Study the drawing (mm; zero at the part's minimum x, y, z) and answer. Coordinates: 2 decimals unless noted, no trailing zeros. Loops run counter-clockwise (first coordinate to the right, second up) from the corner with the lowest first, then second, coordinate; pieces in that order, holes last. Notation, with made-up numbers: (-6, 82) - (52, 82) arc R6 ccw to (52, 92) - close; hole circle Ø11 at (78.25, -37). An arc over 180 degrees is marked (long way). Write each question's results on one line, items separated by ' | '. Start each with the question number.
(1) Find section C-C on z = 2.55. Determine the outline of the cut face in (x, y), then the cut area to 3 significant figures.
(2) Consider line 1 (Y direction, x = 55, z = 1.4); line 2 (X direction, y = 27, z = 4.55); line 3 (Z direction, x = 57.5, y = 53). Determine where each line is inside the solid, lowest interval first. Write a range as from..to.
(3) Find section A-A on y = 16. Determine the outline of the cut face in (x, z), then the cut area to 3 significant figures.
(4) Find section D-D on x = 26. Determine the outline of the cut face in (y, z).
(5) Find section B-B on x = 4.5. Determine the outline of the cut face in (y, z), then the cut area to 3 significant figures.
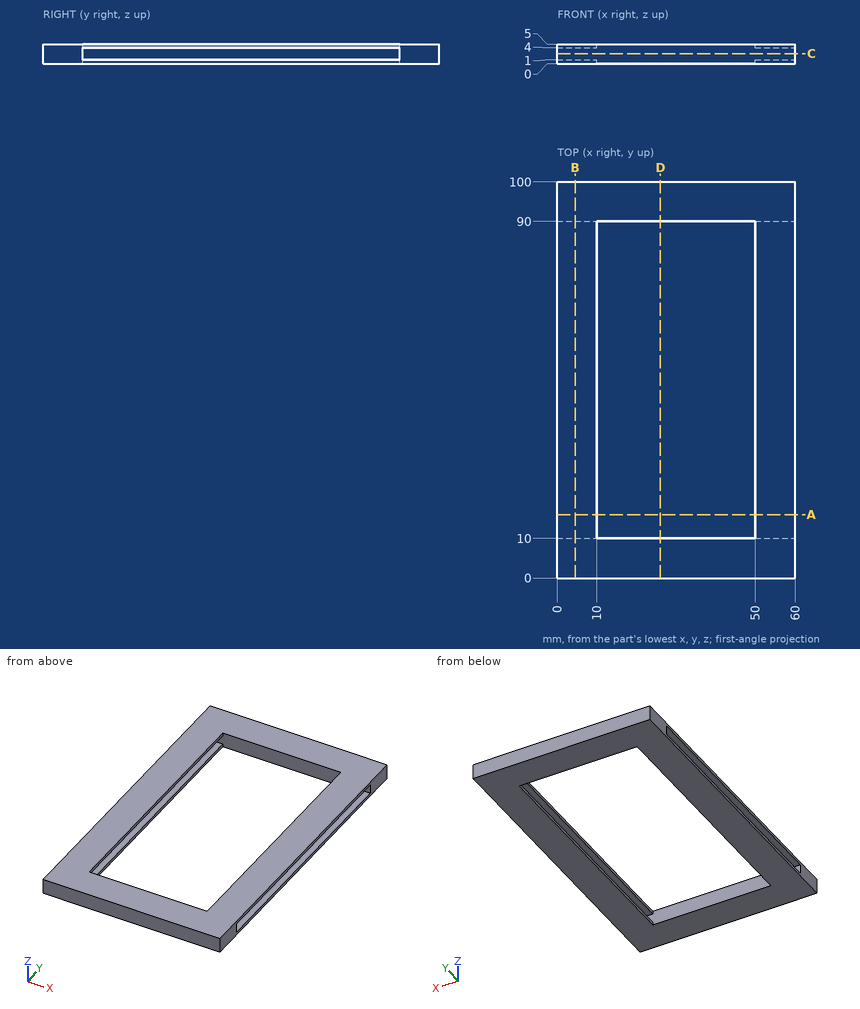
Values:
1) outline: (0, 0) - (60, 0) - (60, 10) - (0, 10) - close; (0, 90) - (60, 90) - (60, 100) - (0, 100) - close | area: 1,200 mm²
2) line 1: y = 0..10, 90..100 | line 2: x = 0..10, 50..60 | line 3: z = 0..1, 4..5
3) outline: (0, 0) - (10, 0) - (10, 1) - (0, 1) - close; (0, 4) - (10, 4) - (10, 5) - (0, 5) - close; (50, 0) - (60, 0) - (60, 1) - (50, 1) - close; (50, 4) - (60, 4) - (60, 5) - (50, 5) - close | area: 40.0 mm²
4) outline: (0, 0) - (10, 0) - (10, 5) - (0, 5) - close; (90, 0) - (100, 0) - (100, 5) - (90, 5) - close
5) outline: (0, 0) - (100, 0) - (100, 5) - (0, 5) - close; hole (10, 1) - (90, 1) - (90, 4) - (10, 4) - close | area: 260 mm²
